```python
from build123d import *

# Parameters (mm, degrees)
SKETCH_1_R               = 2.55
EXTRUDE_1_DEPTH          = 6
SKETCH_7_R               = 11
SKETCH_7_R_2             = 2.55
CUT_EXTRUDE_1_DEPTH      = 14
CUT_EXTRUDE_1_DEPTH_BACK = 5
SKETCH_8_R               = 11
SKETCH_8_R_2             = 2.55
CUT_EXTRUDE_2_DEPTH      = 11
CUT_EXTRUDE_2_DEPTH_BACK = 5
EXTRUDE_2_DEPTH          = 6
SKETCH_3_R               = 2.1
SKETCH_3_W               = 7
SKETCH_3_H               = 6
CUT_EXTRUDE_12_DEPTH     = 7
EXTRUDE_21_DEPTH         = 6
SKETCH_31_R              = 2.1
SKETCH_31_W              = 7
SKETCH_31_H              = 6
CUT_EXTRUDE_13_DEPTH     = 7
EXTRUDE_22_DEPTH         = 6
SKETCH_32_R              = 2.1
SKETCH_32_W              = 7
SKETCH_32_H              = 6
CUT_EXTRUDE_14_DEPTH     = 7
EXTRUDE_23_DEPTH         = 6
SKETCH_33_R              = 2.1
SKETCH_33_W              = 7
SKETCH_33_H              = 6
CUT_EXTRUDE_15_DEPTH     = 7
EXTRUDE_24_DEPTH         = 6
SKETCH_34_R              = 2.1
SKETCH_34_W              = 7
SKETCH_34_H              = 6
CUT_EXTRUDE_16_DEPTH     = 7


with BuildPart() as part:
    # Эскиз1 → Бобышка-Вытянуть1 (new body)
    with BuildSketch(Plane(origin=(0, 0, 0), x_dir=(1, 0, 0), z_dir=(0, 1, 0))):
        with BuildLine():
            Line((-322.202898551, -260), (-322.202898551, -120))
            Line((-322.202898551, -120), (189.797101449, -120))
            Line((189.797101449, -120), (189.797101449, -260))
            Line((189.797101449, -260), (153.844946536, -260))
            ThreePointArc((153.844946536, -260), (151.691579542, -259.600268796), (149.825135208, -258.454336863))
            Line((149.825135208, -258.454336863), (64.602941314, -181.545663137))
            ThreePointArc((64.602941314, -181.545663137), (62.73649698, -180.399731204), (60.583129986, -180))
            Line((60.583129986, -180), (-192.988927088, -180))
            ThreePointArc((-192.988927088, -180), (-195.142294082, -180.399731204), (-197.008738416, -181.545663137))
            Line((-197.008738416, -181.545663137), (-282.230932309, -258.454336863))
            ThreePointArc((-282.230932309, -258.454336863), (-284.097376643, -259.600268796), (-286.250743637, -260))
            Line((-286.250743637, -260), (-322.202898551, -260))
        make_face()
        with Locations((-293.202898551, -210)):
            Circle(SKETCH_1_R, mode=Mode.SUBTRACT)
        with Locations((160.797101449, -210)):
            Circle(SKETCH_1_R, mode=Mode.SUBTRACT)
    extrude(amount=EXTRUDE_1_DEPTH)

    # Эскиз7 → Вырез-Вытянуть1 (cut, two sides)
    with BuildSketch(Plane(origin=(0, 0, 0), x_dir=(1, 0, 0), z_dir=(0, 1, 0))) as cut_extrude_1_sk:
        with Locations((-293.202898551, -240)):
            Circle(SKETCH_7_R)
        with Locations((-280.298199794, -227.095301243)):
            Circle(SKETCH_7_R_2)
        with Locations((-306.107597307, -252.904698757)):
            Circle(SKETCH_7_R_2)
    extrude(amount=CUT_EXTRUDE_1_DEPTH, mode=Mode.SUBTRACT)
    extrude(cut_extrude_1_sk.sketch, amount=-CUT_EXTRUDE_1_DEPTH_BACK, mode=Mode.SUBTRACT)

    # Эскиз8 → Вырез-Вытянуть2 (cut, two sides)
    with BuildSketch(Plane(origin=(0, 0, 0), x_dir=(1, 0, 0), z_dir=(0, 1, 0))) as cut_extrude_2_sk:
        with Locations((160.797101449, -240)):
            Circle(SKETCH_8_R)
        with Locations((147.892402692, -227.095301243)):
            Circle(SKETCH_8_R_2)
        with Locations((173.701800206, -252.904698757)):
            Circle(SKETCH_8_R_2)
    extrude(amount=CUT_EXTRUDE_2_DEPTH, mode=Mode.SUBTRACT)
    extrude(cut_extrude_2_sk.sketch, amount=-CUT_EXTRUDE_2_DEPTH_BACK, mode=Mode.SUBTRACT)

    # Эскиз2 → Бобышка-Вытянуть2 (add)
    with BuildSketch(Plane(origin=(139.797101449, 0, 243), x_dir=(0, 0, 1), z_dir=(0, 1, 0))):
        with BuildLine():
            Line((13, 53), (-13, 53))
            ThreePointArc((-13, 53), (-14.118033989, 52.736067977), (-15, 52))
            Line((-15, 52), (-16.2, 50.4))
            ThreePointArc((-16.2, 50.4), (-16.552786405, 50.105572809), (-17, 50))
            Line((-17, 50), (17, 50))
            ThreePointArc((17, 50), (16.552786405, 50.105572809), (16.2, 50.4))
            Line((16.2, 50.4), (15, 52))
            ThreePointArc((15, 52), (14.118033989, 52.736067977), (13, 53))
        make_face()
    extrude(amount=EXTRUDE_2_DEPTH)

    # Эскиз3 → Вырез-Вытянуть12 (cut, through all)
    with BuildSketch(Plane(origin=(139.797101449, 6, 243), x_dir=(0, 0, 1), z_dir=(0, 1, 0))):
        with Locations((0, 47)):
            Circle(SKETCH_3_R)
        with Locations((9.531849908, 47)):
            Rectangle(SKETCH_3_W, SKETCH_3_H)
        with Locations((-9.531849908, 47)):
            Rectangle(SKETCH_3_W, SKETCH_3_H)
    extrude(amount=-CUT_EXTRUDE_12_DEPTH, mode=Mode.SUBTRACT)

    # Эскиз21 → Бобышка-Вытянуть21 (add)
    with BuildSketch(Plane(origin=(139.797101449, 0, 137), x_dir=(0, 0, 1), z_dir=(0, 1, 0))):
        with BuildLine():
            Line((13, 53), (-13, 53))
            ThreePointArc((-13, 53), (-14.118033989, 52.736067977), (-15, 52))
            Line((-15, 52), (-16.2, 50.4))
            ThreePointArc((-16.2, 50.4), (-16.552786405, 50.105572809), (-17, 50))
            Line((-17, 50), (17, 50))
            ThreePointArc((17, 50), (16.552786405, 50.105572809), (16.2, 50.4))
            Line((16.2, 50.4), (15, 52))
            ThreePointArc((15, 52), (14.118033989, 52.736067977), (13, 53))
        make_face()
    extrude(amount=EXTRUDE_21_DEPTH)

    # Эскиз31 → Вырез-Вытянуть13 (cut, through all)
    with BuildSketch(Plane(origin=(139.797101449, 6, 137), x_dir=(0, 0, 1), z_dir=(0, 1, 0))):
        with Locations((0, 47)):
            Circle(SKETCH_31_R)
        with Locations((9.531849908, 47)):
            Rectangle(SKETCH_31_W, SKETCH_31_H)
        with Locations((-9.531849908, 47)):
            Rectangle(SKETCH_31_W, SKETCH_31_H)
    extrude(amount=-CUT_EXTRUDE_13_DEPTH, mode=Mode.SUBTRACT)

    # Эскиз22 → Бобышка-Вытянуть22 (add)
    with BuildSketch(Plane(origin=(-272.202898551, 0, 243), x_dir=(0, 0, -1), z_dir=(0, 1, 0))):
        with BuildLine():
            Line((13, 53), (-13, 53))
            ThreePointArc((-13, 53), (-14.118033989, 52.736067977), (-15, 52))
            Line((-15, 52), (-16.2, 50.4))
            ThreePointArc((-16.2, 50.4), (-16.552786405, 50.105572809), (-17, 50))
            Line((-17, 50), (17, 50))
            ThreePointArc((17, 50), (16.552786405, 50.105572809), (16.2, 50.4))
            Line((16.2, 50.4), (15, 52))
            ThreePointArc((15, 52), (14.118033989, 52.736067977), (13, 53))
        make_face()
    extrude(amount=EXTRUDE_22_DEPTH)

    # Эскиз32 → Вырез-Вытянуть14 (cut, through all)
    with BuildSketch(Plane(origin=(-272.202898551, 6, 243), x_dir=(0, 0, -1), z_dir=(0, 1, 0))):
        with Locations((0, 47)):
            Circle(SKETCH_32_R)
        with Locations((9.531849908, 47)):
            Rectangle(SKETCH_32_W, SKETCH_32_H)
        with Locations((-9.531849908, 47)):
            Rectangle(SKETCH_32_W, SKETCH_32_H)
    extrude(amount=-CUT_EXTRUDE_14_DEPTH, mode=Mode.SUBTRACT)

    # Эскиз23 → Бобышка-Вытянуть23 (add)
    with BuildSketch(Plane(origin=(-272.202898551, 0, 137), x_dir=(0, 0, -1), z_dir=(0, 1, 0))):
        with BuildLine():
            Line((13, 53), (-13, 53))
            ThreePointArc((-13, 53), (-14.118033989, 52.736067977), (-15, 52))
            Line((-15, 52), (-16.2, 50.4))
            ThreePointArc((-16.2, 50.4), (-16.552786405, 50.105572809), (-17, 50))
            Line((-17, 50), (17, 50))
            ThreePointArc((17, 50), (16.552786405, 50.105572809), (16.2, 50.4))
            Line((16.2, 50.4), (15, 52))
            ThreePointArc((15, 52), (14.118033989, 52.736067977), (13, 53))
        make_face()
    extrude(amount=EXTRUDE_23_DEPTH)

    # Эскиз33 → Вырез-Вытянуть15 (cut, through all)
    with BuildSketch(Plane(origin=(-272.202898551, 6, 137), x_dir=(0, 0, -1), z_dir=(0, 1, 0))):
        with Locations((0, 47)):
            Circle(SKETCH_33_R)
        with Locations((9.531849908, 47)):
            Rectangle(SKETCH_33_W, SKETCH_33_H)
        with Locations((-9.531849908, 47)):
            Rectangle(SKETCH_33_W, SKETCH_33_H)
    extrude(amount=-CUT_EXTRUDE_15_DEPTH, mode=Mode.SUBTRACT)

    # Эскиз24 → Бобышка-Вытянуть24 (add)
    with BuildSketch(Plane(origin=(-66.202898551, 0, 130), x_dir=(-1, 0, 0), z_dir=(0, 1, 0))):
        with BuildLine():
            Line((13, 53), (-13, 53))
            ThreePointArc((-13, 53), (-14.118033989, 52.736067977), (-15, 52))
            Line((-15, 52), (-16.2, 50.4))
            ThreePointArc((-16.2, 50.4), (-16.552786405, 50.105572809), (-17, 50))
            Line((-17, 50), (17, 50))
            ThreePointArc((17, 50), (16.552786405, 50.105572809), (16.2, 50.4))
            Line((16.2, 50.4), (15, 52))
            ThreePointArc((15, 52), (14.118033989, 52.736067977), (13, 53))
        make_face()
    extrude(amount=EXTRUDE_24_DEPTH)

    # Эскиз34 → Вырез-Вытянуть16 (cut, through all)
    with BuildSketch(Plane(origin=(-66.202898551, 6, 130), x_dir=(-1, 0, 0), z_dir=(0, 1, 0))):
        with Locations((0, 47)):
            Circle(SKETCH_34_R)
        with Locations((9.531849908, 47)):
            Rectangle(SKETCH_34_W, SKETCH_34_H)
        with Locations((-9.531849908, 47)):
            Rectangle(SKETCH_34_W, SKETCH_34_H)
    extrude(amount=-CUT_EXTRUDE_16_DEPTH, mode=Mode.SUBTRACT)


solid = part.part
```
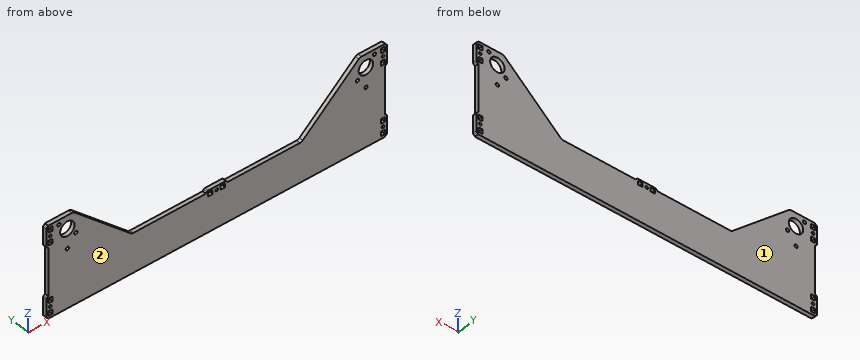
Build history of the part. All positions in model axes, mm. Face numbers are marked on the shaded views. Round coordinates to 2 decimals unless told otherwise and drop trailing zeros.
1) Mould opens along Y. For the marked faces 1 and 2 say: +Y half, -Y half, draft (parallel to the pull), parting line (faces both ways), or undercut.
2) Band-saw the part on A-A, the plane y = 2.25. Give the number of separate pieces and of enclosed holes in the cut face, and give its area (3 significant figures).
3) Pin check, flat tips, straight feed: pin 1 (1 mm diameter, centred on y = 5, z = 183.5, fed in from -X); pin 2 (2.5 mm diameter, centred on x = 186.8, z = 137, fed in from +Y); pin 3 (2 mm diameter, centred on x = 106.5, y = 1, fed in from +Z). Stop position of each tip, or through.
4) Drill centre lines: probe 1 along X at (y, z) = (3.2, 177); probe 2 along X at (y, z) = (2.9, 126); probe 3 along Z at (x, y) = (-66, 1.6). Where is each one in solid material? Low to high.
Ans:
1. face 1: +Y half
1. face 2: -Y half
2. separate pieces: 1
2. enclosed holes: 23
2. area: 43,000 mm2
3. pin 1: stops at x = -322.2
3. pin 2: passes through
3. pin 3: stops at z = 220.26
4. probe 1: x = -322.2 to -79.23, -72.23 to -68.3, -64.1 to -60.17, -53.17 to 189.8
4. probe 2: x = -325.2 to -322.2, -316.2 to 183.8, 189.8 to 192.8
4. probe 3: z = 120 to 174.91, 179.09 to 183
